```python
from build123d import *

# Parameters (mm, degrees)
BOSS_EXTRUDE1_DEPTH = 2
FILLET1_R           = 2


with BuildPart() as part:
    # Sketch1 → Boss-Extrude1 (new body)
    with BuildSketch(Plane.XY):
        Polygon((-45, 7), (-55, 2.5), (-105, 2.5), (-113, 0), (-105, -2.5), (-55, -2.5), (-45, -7), (45, -7), (45, 7), align=None)
    extrude(amount=BOSS_EXTRUDE1_DEPTH)

    # Fillet1
    fillet1_edges = [part.edges().sort_by_distance(p)[0] for p in [
        (45, -7, 1),
        (45, 7, 1),
    ]]
    fillet(fillet1_edges, radius=FILLET1_R)


solid = part.part
```
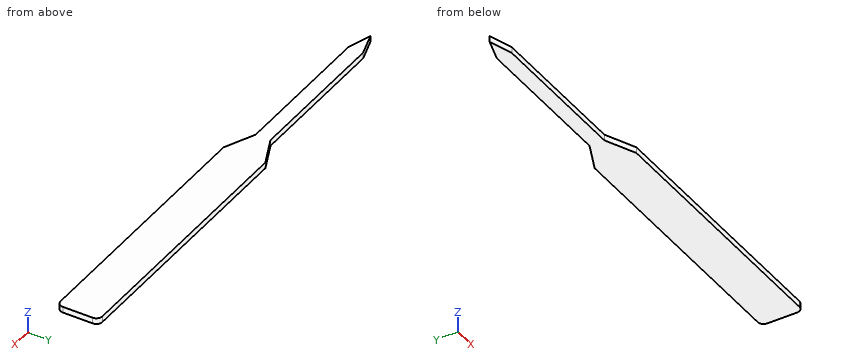
Here's how the part is built. I have some questions about the finished solid (model axes, mm). Coordinates: 2 decimals unless noted, no trailing zeros. Loops run counter-clockwise (first coordinate to the right, second up) from the corner with the lowest first, then second, coordinate; pieces in that order, holes last. Notation, with made-up numbers: M 27,73.25 L 57,73.25 A16 cw 57,89.25 Z; hole C -4,39.25 d6. An arc over 180 degrees is marked long. One line per item, written item: value.
1. Imagine slicing it at B-B (x = -83). List the corners of the cut face in (y, z) for me.
Geometry says:
outline: M -2.5,0 L 2.5,0 L 2.5,2 L -2.5,2 Z
2. Will these pins go through, and if not, where does the flat tip stop? pin 1 Ø1 at (x, z) = (-68.5, 1.5) entering from -Y; pin 2 Ø1 at (x, z) = (-70, 0.5) entering from +Y.
Geometry says:
pin 1: stops at y = -2.5
pin 2: stops at y = 2.5
3. Imagine slicing it at A-A (z = 1.4). List the corners of the cut face in (x, y) for me.
Geometry says:
outline: M -113,0 L -105,-2.5 L -55,-2.5 L -45,-7 L 43,-7 A2 ccw 45,-5 L 45,5 A2 ccw 43,7 L -45,7 L -55,2.5 L -105,2.5 Z
4. Please list where these lines run through material, in increasing order: probe 1 along Y at (x, z) = (-67.5, 0.4); probe 2 along X at (y, z) = (-6, 1.1); probe 3 along X at (y, z) = (3.75, 0.7).
Geometry says:
probe 1: y = -2.5 to 2.5
probe 2: x = -47.22 to 44.73
probe 3: x = -52.22 to 45
